Check sheet for the modelled part. Datum: model origin and axes. Units: mm. Give positions to 0.01 mm unless a question says otherwise; leave off trailing zeros. Write each loop counter-clockwise with the first axis right and the second up, starting at its lowest first coordinate (ties: lowest second). Pieces come first, ordered by that corner, then holes. Notation, with made-up numbers: M -33.5,-23.5 L 19.5,-23.5 A23 cw 19.5,-12.5 Z; hole C 3.5,34.5 d7. An arc over 180 degrees is marked long. One line per item, written item: value. Start each with the question number.
Autodesk Inventor part; units mm, degrees
ref_plane "YZ Plane" through (0, 0, 0) normal (1, 0, 0) x (0, 1, 0)
ref_plane "XZ Plane" through (0, 0, 0) normal (0, 1, 0) x (-1, 0, 0)
ref_plane "XY Plane" through (0, 0, 0) normal (0, 0, 1) x (1, 0, 0)
sketch "Sketch1" plane through (0, 0, 0) normal (0, 1, 0) x (-1, 0, 0)
  circle A0 centre (0, 12.1747) radius 12.108
  arc A1 (7.1431, 10.8771) -> (-7.6488, 10.8771) centre (-0.2529, 11.8554) ccw
  point P0 (0, 0)
extrude "Extrusion1" add sketch "Sketch1" along normal blind 5
sketch "Sketch2" plane through (0, 0, 12.1747) normal (0, -1, 0) x (1, 0, 0)
  point P0 (0, -12.1747)
sketch "Sketch3" plane through (0, 5, 12.1747) normal (0, 1, 0) x (1, 0, 0)
  point P0 (0, 12.1747)
sketch "Sketch4" plane through (0, 0, 0) normal (0, 1, 0) x (-1, 0, 0)
  arc A0 (2.5285, 18.8375) -> (2.5917, 4.9938) centre (-0.8103, 11.9003) ccw
  point P0 (0, 0)
scale "Scale1" factors (5, 5, 5) then translate (0, 0, -48.6988) bodies 1
scale "Scale2" factors (2, 2, 2) then translate (0, 0, -12.1747) bodies 1
properties part number "drum"
1) Gauge pin test, flat ends, axial feed: pin 1 (8 mm diameter, centred on x = 16, y = 6, fed in from -Z); pin 2 (10 mm diameter, centred on y = 38.5, z = 6, fed in from -X); pin 3 (2 mm diameter, centred on y = 8, z = 70.5, fed in from +X); pin 4 (12 mm diameter, centred on x = -10.5, z = 91.5, fed in from -Y). Record the tip position at first contact, or that the pin passes through.
2) Material ranges on L1, parallel to Z at x = 0.5, y = 33; L2, parallel to X at y = 29.5, z = 73; L3, parallel to X at y = 13, z = -33, recorded low to high. Write a range as from..to.
3) Cross-section at C-C (z = -84.5). Record the boundary of the cut face in (x, y), plus the area to 3 significant figures.
4) Cross-section at A-A (x = -33.5). Record the boundary of the cut face in (y, z).
5) Cross-section at B-B (y = 32.5). Record the boundary of the cut face in (x, z), plus the area to 3 significant figures.
Data:
1. pin 1: stops at z = -108.31
1. pin 2: stops at x = -121.07
1. pin 3: stops at x = 106.65
1. pin 4: stops at y = 0
2. L1: z = -108.9..133.25
2. L2: x = -104.69..104.69
2. L3: x = -112.34..112.34
3. outline: M -72.9,0 L 72.9,0 L 72.9,50 L -72.9,50 Z
3. area: 7,290 mm2
4. outline: M 0,-104.18 L 50,-104.18 L 50,128.53 L 0,128.53 Z
5. outline: C 0,12.17 d242.16
5. area: 46,100 mm2
